```python
from build123d import *

# Parameters (mm, degrees)
F1_DEPTH = 10
F2_D     = 12


with BuildPart() as f1:
    # F0 (on Front) → F1 (new body)
    with BuildSketch(Plane.XZ):
        with BuildLine():
            ThreePointArc((0, 40), (-20, 20), (0, 0))
            Line((0, 0), (60, 0))
            ThreePointArc((60, 0), (80, 20), (60, 40))
            Line((60, 40), (0, 40))
        make_face()
    extrude(amount=F1_DEPTH)

    # F2 (through all)
    with Locations(Plane(origin=(0, 0, 0), x_dir=(1, 0, 0), z_dir=(0, 1, 0))):
        with Locations((0, -20), (60, -20)):
            Hole(F2_D / 2)


solid = f1.part
```
Verification items for the finished model (mm, model axes). Give positions to 0.01 mm unless a question says otherwise; leave off trailing zeros. Order: outer loops, then holes, each group sorted by start corner. A loop starts at its lowest first (then second) coordinate and runs counter-clockwise, first axis right, second up. Notation, with made-up numbers: (62.5, 36.5) - (111.5, 36.5) arc R16 cw to (111.5, 53.5) - close; hole circle Ø10 at (80.25, 89). An arc over 180 degrees is marked (long way). Answer as CSV lines item,"result". Start each with the question number.
Item 1: Gauge pin test, flat ends, axial feed: pin 1 (5 mm diameter, centred on x = 35.5, y = -5.5, fed in from -Z); pin 2 (11 mm diameter, centred on x = 60, z = 20, fed in from -Y); pin 3 (2 mm diameter, centred on y = -4.5, z = 9, fed in from -X). Record the tip position at first contact, or that the pin passes through.
Item 2: Mould release check, pull along X, two halves, no side actions. Record for faces 1 (the face through (0.78, -5.07, 14.05)), 2 (the face through (30, -5, 0)), 3 (the face through (-20, -5, 20)): released by +X, released by -X, zero draft, split by the parting line, or undercut.
Item 3: Section check D-D, the plane x = 67.5. Record the boundary of the cut face in (y, z).
Item 4: Section check C-C, the plane z = 8. Record the boundary of the cut face in (x, y).
Item 5: Section check B-B, the plane y = -5.5. Record the boundary of the cut face in (x, z).
Item 6: Material ranges on L1, parallel to X at y = -2, z = 20; L2, parallel to Z at x = 60, y = -7.75; L3, parallel to X at y = -5, z = 23.5, recorded low to high.
Item 7: Section check A-A, the plane z = 20. Record the boundary of the cut face in (x, y).
Filled in:
1,pin 1,"z = 0"
1,pin 2,"through"
1,pin 3,"x = -17.32"
2,face 1,"undercut"
2,face 2,"zero draft"
2,face 3,"released by -X"
3,outline,"(-10, 1.46) - (0, 1.46) - (0, 38.54) - (-10, 38.54) - close"
4,outline,"(-16, -10) - (76, -10) - (76, 0) - (-16, 0) - close"
5,outline,"(0, 0) - (60, 0) arc R20 ccw to (60, 40) - (0, 40) arc R20 ccw to start; hole circle Ø12 at (0, 20); hole circle Ø12 at (60, 20)"
6,L1,"-20 to -6, 6 to 54, 66 to 80"
6,L2,"0 to 14, 26 to 40"
6,L3,"-19.69 to -4.87, 4.87 to 55.13, 64.87 to 79.69"
7,outline,"(-20, -10) - (-6, -10) - (-6, 0) - (-20, 0) - close; (6, -10) - (54, -10) - (54, 0) - (6, 0) - close; (66, -10) - (80, -10) - (80, 0) - (66, 0) - close"
